```python
from build123d import *

# Parameters (mm, degrees)
PAD_DEPTH       = 45
SKETCH008_R     = 11.2
SKETCH008_R_2   = 10.8
POCKET_DEPTH    = 38.001
SKETCH009_R     = 2.7
POCKET001_DEPTH = 40.001
SKETCH010_R     = 4.7
POCKET002_DEPTH = 5
POCKET003_DEPTH = 4
SKETCH011_W     = 2
SKETCH011_H     = 32
POCKET004_DEPTH = 37.8
FILLET_R        = 2


with BuildPart() as part:
    # Sketch → Pad (new body)
    with BuildSketch(Plane.XY):
        with BuildLine():
            Line((-16, 19), (16, 19))
            ThreePointArc((20, 15), (18.828427, 17.828427), (16, 19))
            Line((20, 15), (20, -15))
            ThreePointArc((16, -19), (18.828427, -17.828427), (20, -15))
            Line((16, -19), (-16, -19))
            ThreePointArc((-20, -15), (-18.828427, -17.828427), (-16, -19))
            Line((-20, -15), (-20, 15))
            ThreePointArc((-16, 19), (-18.828427, 17.828427), (-20, 15))
        make_face()
    extrude(amount=PAD_DEPTH)

    # Sketch008 → Pocket (cut, through all)
    with BuildSketch(Plane(origin=(0, 19, 0), x_dir=(-1, 0, 0), z_dir=(0, 1, 0))):
        with Locations((0, 38.034691)):
            Circle(SKETCH008_R)
        with Locations((0, 6.5)):
            Circle(SKETCH008_R_2)
    extrude(amount=-POCKET_DEPTH, mode=Mode.SUBTRACT)

    # Sketch009 → Pocket001 (cut, through all)
    with BuildSketch(Plane.YZ.offset(20)):
        with Locations((0, 23)):
            Circle(SKETCH009_R)
    extrude(amount=-POCKET001_DEPTH, mode=Mode.SUBTRACT)

    # Sketch010 → Pocket002 (cut)
    with BuildSketch(Plane.YZ.offset(20)):
        with Locations((0, 23)):
            Circle(SKETCH010_R)
    extrude(amount=-POCKET002_DEPTH, mode=Mode.SUBTRACT)

    # Sketch002 → Pocket003 (cut)
    with BuildSketch(Plane(origin=(-20, 0, 0), x_dir=(0, -1, 0), z_dir=(-1, 0, 0))):
        Polygon((4.156922, 23), (2.078461, 26.6), (-2.078461, 26.6), (-4.156922, 23), (-2.078461, 19.4), (2.078461, 19.4), align=None)
    extrude(amount=-POCKET003_DEPTH, mode=Mode.SUBTRACT)

    # Sketch011 → Pocket004 (cut)
    with BuildSketch(Plane.XZ.offset(19)):
        with Locations((0, 16)):
            Rectangle(SKETCH011_W, SKETCH011_H)
    extrude(amount=-POCKET004_DEPTH, mode=Mode.SUBTRACT)

    # Fillet
    fillet_edges = [part.edges().sort_by_distance(p)[0] for p in [
        (20, 0, 0),
        (20, 0, 45),
        (-20, 0, 0),
        (-20, 0, 45),
    ]]
    fillet(fillet_edges, radius=FILLET_R)


solid = part.part
```
Build history of the part. All positions in model axes, mm. A direction names the side the tool comes from. Coordinates: 2 decimals unless noted, no trailing zeros. Write each loop counter-clockwise with the first axis right and the second up, starting at its lowest first coordinate (ties: lowest second). Pieces come first, ordered by that corner, then holes.
1. Band-saw the part on D-D, the plane y = -14. Give the cut face in (x, z).
Answer block:
outline: (-20, 2) arc R2 ccw to (-18, 0) - (-8.62, 0) arc R10.8 cw to (-1, 17.25) - (-1, 26.88) arc R11.2 cw to (-8.77, 45) - (-18, 45) arc R2 ccw to (-20, 43) - close; (1, 17.25) arc R10.8 cw to (8.62, 0) - (18, 0) arc R2 ccw to (20, 2) - (20, 43) arc R2 ccw to (18, 45) - (8.77, 45) arc R11.2 cw to (1, 26.88) - close
2. Band-saw the part on A-A, the plane z = 13. Give the cut face in (x, y).
Answer block:
outline: (-20, -15) arc R4 ccw to (-16, -19) - (-8.62, -19) - (-8.62, 19) - (-16, 19) arc R4 ccw to (-20, 15) - close; (8.62, -19) - (16, -19) arc R4 ccw to (20, -15) - (20, 15) arc R4 ccw to (16, 19) - (8.62, 19) - close
3. Band-saw the part on B-B, the plane x = -12. Give the cut face in (y, z), and give its area (3 significant figures).
Answer block:
outline: (-19, 2) arc R2 ccw to (-17, 0) - (17, 0) arc R2 ccw to (19, 2) - (19, 43) arc R2 ccw to (17, 45) - (-17, 45) arc R2 ccw to (-19, 43) - close; hole circle Ø5.4 at (0, 23)
area: 1,680 mm2
4. 3-axis set-ups, long thin cutter, end or side, ignore diameter. For faces 5 (the flat face through (1, 0, 20)), 6 (the flat face through (-18, -3, 25)), 7 (the flat face through (15, 2.02, 20.98)): which of +Z, -Z, +X, -X, +Y, -Y reach the whole face in a straight line?
Answer block:
face 5: +Z, -Z, -Y
face 6: -X
face 7: +X
5. Drill centre lines: probe 1 along X at (y, z) = (14.5, 19.5); probe 2 along X at (y, z) = (0, 7); probe 3 along Z at (x, y) = (4, 0). Where is each one in solid material? Low to high.
Answer block:
probe 1: x = -20 to -1, 1 to 20
probe 2: x = -20 to -10.79, 10.79 to 20
probe 3: z = 16.53 to 20.3, 25.7 to 27.57
6. Band-saw the part on C-C, the plane y = 0. Give the number of separate pieces and of enclosed holes in the cut face, and give its area (3 significant figures).
Answer block:
separate pieces: 4
enclosed holes: 0
area: 888 mm2
7. Drop flat-ended pins along their axis: pin 1 (3 mm diameter, centred on x = -2, y = 9.5, fed in from -Z); pin 2 (3.5 mm diameter, centred on y = 1.5, z = 23.5, fed in from -X); pin 3 (13.5 mm diameter, centred on x = 0, z = 38.03, fed in from -Y); pin 4 (3 mm diameter, centred on y = 2, z = 21.5, fed in from +X). Give the stop position or say it passes through.
Answer block:
pin 1: stops at z = 16.72
pin 2: stops at x = -16
pin 3: passes through
pin 4: stops at x = 15
8. Pull direction Y, two halves, no side cores. Call faces 1 (the flat face through (-13, 0, 45)), 2 (the cylindrical face through (-12.26, 18.4, 0.57)), 3 (the flat face through (-18, 0, 26.6)), 4 (the cylindrical face through (-18.859, -17.797, 22.213)): released by +Y, released by -Y, zero draft, split by the parting line, or undercut.
Answer block:
face 1: zero draft
face 2: released by +Y
face 3: undercut
face 4: released by -Y
